```python
from build123d import *

# Parameters (mm, degrees)
SKETCH_1_R      = 28
SKETCH_1_R_2    = 7
EXTRUDE_1_DEPTH = 25


with BuildPart() as part:
    # 草图1 → 凸台-拉伸1 (new body)
    with BuildSketch(Plane(origin=(0, 0, 0), x_dir=(1, 0, 0), z_dir=(0, 1, 0))):
        with BuildLine():
            Line((150, 28), (-150, 28))
            ThreePointArc((-150, 28), (-130.201010127, 19.798989873), (-122, 0))
            ThreePointArc((-122, 0), (-130.201010127, -19.798989873), (-150, -28))
            Line((-150, -28), (150, -28))
            ThreePointArc((150, -28), (122, 0), (150, 28))
        make_face()
        with Locations((150, 0)):
            Circle(SKETCH_1_R)
        with Locations((150, 0)):
            Circle(SKETCH_1_R_2, mode=Mode.SUBTRACT)
        with Locations((-150, 0)):
            Circle(SKETCH_1_R)
        with Locations((-150, 0)):
            Circle(SKETCH_1_R_2, mode=Mode.SUBTRACT)
    extrude(amount=EXTRUDE_1_DEPTH)


solid = part.part
```
Input: part model. Units: mm. Frame: model coordinates. Coordinates: 2 decimals unless noted, no trailing zeros. Order: outer loops, then holes, each group sorted by start corner. A loop starts at its lowest first (then second) coordinate and runs counter-clockwise, first axis right, second up. Notation, with made-up numbers: (89.5, -14.75) - (102.5, -14.75) arc R35 cw to (102.5, 18.25) - close; hole circle Ø11 at (13, -33). An arc over 180 degrees is marked (long way). Return JSON: item names as keys, results as strings.
Q1. Ray query, probe 1 along X at (y, z) = (17, 0); probe 2 along Z at (x, y) = (-150, 7.5); probe 3 along X at (y, z) = (21.5, 16). Return the intervals inside material, ascending.
The answers:
{"probe 1": "x = -178 to -157, -143 to 143, 157 to 178", "probe 2": "z = -28 to -7, 7 to 28", "probe 3": "x = -172.98 to 172.98"}
Q2. Cut plane A-A (z = 0). Return loops of the section in (x, y), then the cut area to 3 significant figures.
The answers:
{"outline": "(-178, 0) - (-157, 0) - (-157, 25) - (-178, 25) - close; (-143, 0) - (143, 0) - (143, 25) - (-143, 25) - close; (157, 0) - (178, 0) - (178, 25) - (157, 25) - close", "area": "8,200 mm2"}
Q3. First-contact query: pin 1 (10 mm diameter, centred on y = 10, z = -5, fed in from +X); pin 2 (11 mm diameter, centred on x = 150, z = 0, fed in from -Y); pin 3 (6 mm diameter, centred on y = 16.5, z = 5.5, fed in from -X). Flat tips, straight axial feed; report the tip coordinate or a pass-through.
The answers:
{"pin 1": "stops at x = 178", "pin 2": "passes through", "pin 3": "stops at x = -177.89"}
Q4. Cut plane B-B (y = 9.25). Return loops of the section in (x, z), then the cut area to 3 significant figures.
The answers:
{"outline": "(-150, -28) - (150, -28) arc R28 ccw to (150, 28) - (-150, 28) arc R28 ccw to start; hole circle Ø14 at (-150, 0); hole circle Ø14 at (150, 0)", "area": "19,000 mm2"}
Q5. Cut plane C-C (z = -23). Return loops of the section in (x, y), then the cut area to 3 significant figures.
The answers:
{"outline": "(-165.97, 0) - (165.97, 0) - (165.97, 25) - (-165.97, 25) - close", "area": "8,300 mm2"}
Q6. Draft query along X for faces 1 (the cylindrical face through (-143.534, 12.325, 2.681)), 2 (the cylindrical face through (177.993, 12.325, 0.616)), 3 (the flat face through (-2, 12, 28)). Return one class per face: +X half, -X half, draft (parallel to the pull), parting line (faces both ways), or undercut.
The answers:
{"face 1": "undercut", "face 2": "+X half", "face 3": "draft"}
